Check sheet for the drawn part. Datum: minimum x, y, z corner. Units: mm. A direction names the side the tool comes from. Coordinates: 2 decimals unless noted, no trailing zeros. Loops run counter-clockwise (first coordinate to the right, second up) from the corner with the lowest first, then second, coordinate; pieces in that order, holes last.
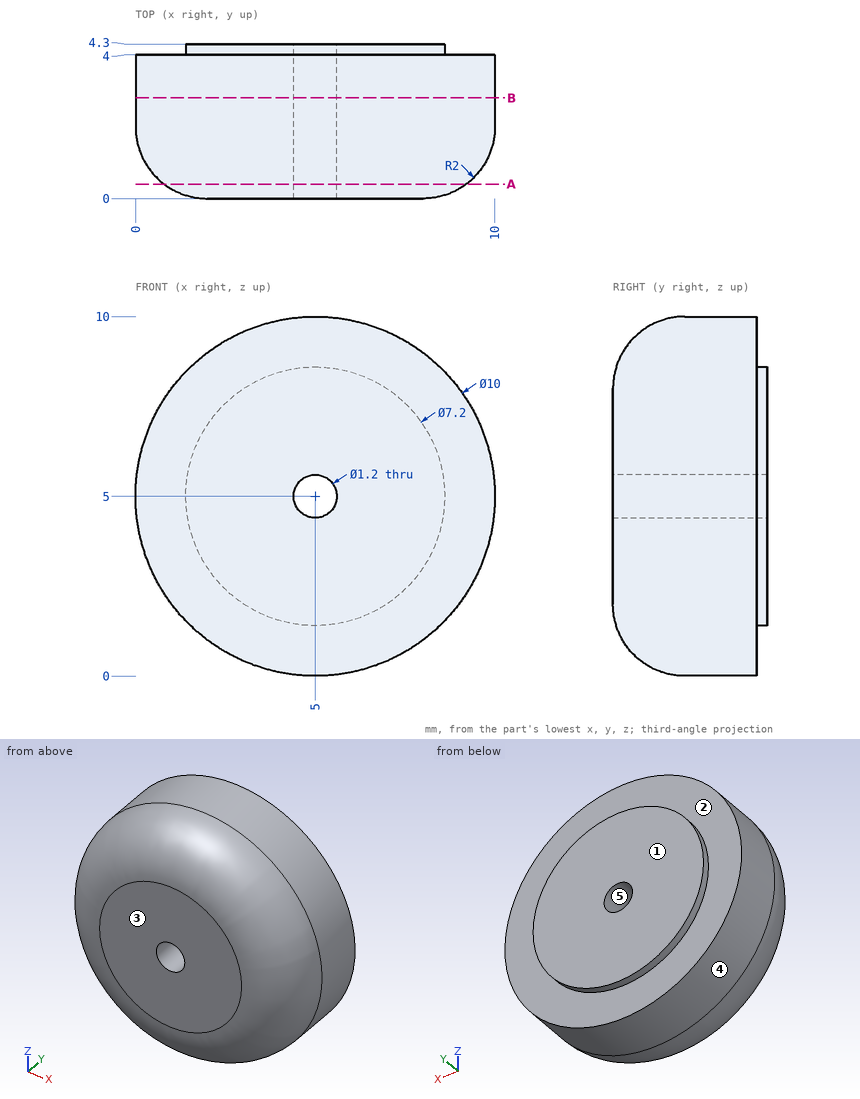
1) Scan lines: line 1 (X direction, y = 2.9, z = 5); line 2 (Z direction, x = 4.5, y = 3.6); line 3 (Z direction, x = 4.75, y = 1.45). Record each from-to range of solid material in increasing order.
Answer sheet:
line 1: x = 0 to 4.4, 5.6 to 10
line 2: z = 0.03 to 4.67, 5.33 to 9.97
line 3: z = 0.08 to 4.45, 5.55 to 9.92
2) Section check A-A on y = 0.4. Enter the section's corners in (x, z), plus the area to 3 significant figures.
Answer sheet:
outline: circle Ø8.4 at (5, 5); hole circle Ø1.2 at (5, 5)
area: 54.3 mm2
3) Depth check by flat-ended pin: pin 1 (1 mm diameter, centred on x = 7.5, z = 3, fed in from -Y); pin 2 (1 mm diameter, centred on x = 7, y = 1.5, fed in from -Z). Enter the tip coordinate at first touch or a pass-through.
Answer sheet:
pin 1: stops at y = 0
pin 2: stops at z = 0.27
4) Mould release check, pull along Z, two halves, no side actions. Record for the marked faces 3, 4 and 5: +Z half, -Z half, draft (parallel to the pull), parting line (faces both ways), or undercut.
Answer sheet:
face 3: draft
face 4: parting line
face 5: undercut
5) Section check B-B on y = 2.8. Enter the section's corners in (x, z).
Answer sheet:
outline: circle Ø10 at (5, 5); hole circle Ø1.2 at (5, 5)
6) Set-up check for the marked faces 1 and 2: record each of +Z, -Z, +X, -X, +Y, -Y from which the full face is reachable in a straight line by a thin tool's end or side.
Answer sheet:
face 1: +Z, -Z, +X, -X, +Y
face 2: +Y
